Can you work these out from the model? Positions are in its coordinate system, mm. Face numbers are marked on the shaded views. A direction names the side the tool comes from. Coordinates: 2 decimals unless noted, no trailing zeros. Order: outer loops, then holes, each group sorted by start corner. A loop starts at its lowest first (then second) coordinate and runs counter-clockwise, first axis right, second up. Notation, with made-up numbers: (-31, 14.25) -> (24, 14.25) arc R16 cw to (24, 21.25) -> close; hole circle Ø9 at (72.5, 71.5). An arc over 180 degrees is marked (long way). Answer as a JSON object with one key per item and string values. Group by question number.
(1) I want a section at A-A, the plane z = 0. List the corners of the cut face in (x, y) for me, plus the area to 3 significant figures.
(2) I want a section at D-D, the plane y = -27. List the corners of the cut face in (x, z) for me, plus the area to 3 significant figures.
(3) I want a section at B-B, the plane x = 0. List the corners of the cut face in (y, z) for me, plus the area to 3 significant figures.
(4) I want a section at C-C, the plane y = -61. List the corners of the cut face in (x, z) for me, plus the area to 3 significant figures.
(5) Which directions (+Z, -Z, +X, -X, +Y, -Y) give clear straight access to the entire face, cutting with the end or side of a thin tool? Please do the marked faces 1 and 2.
(6) For pin 1 (6 mm diameter, centred on x = 5.5, y = -43, fed in from +Z); pin 2 (12 mm diameter, centred on x = 11.5, y = -39.5, fed in from +Z); pin 3 (6 mm diameter, centred on x = 10.5, y = -60, fed in from -Z), each with a flat end and sliding along its axis, tell me the tip position at first contact or that it passes through.
(7) I need wall thicknesses on line 1 (Y direction, x = 0, z = 16.5); line 2 (X direction, y = -38.5, z = -0.5) (3 decimals); line 3 (Z direction, x = 2.5, y = -6). Which ranges of each line are inside material? Lowest first, please.
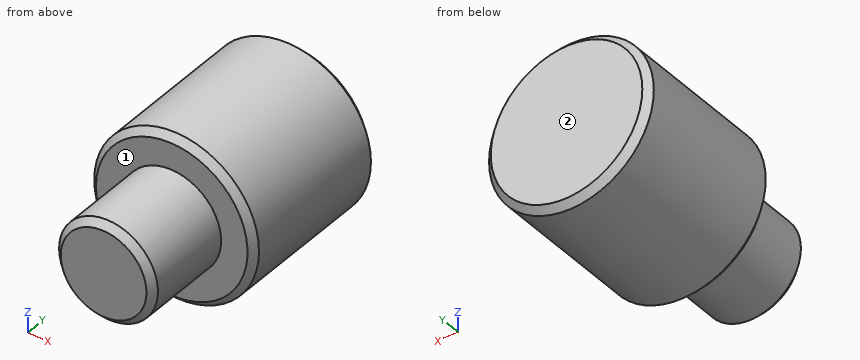
from build123d import *

# Parameters (mm, degrees)
CHAMFER1_SIZE = 2


with BuildPart() as part:
    # Sketch1 → Revolve1 (revolve)
    with BuildSketch(Plane.XY, mode=Mode.PRIVATE) as revolve1_sk:
        Polygon((0, 0), (25, 0), (25, -50), (15, -50), (15, -78), (0, -78), align=None)
    revolve(revolve1_sk.sketch.rotate(Axis((0, 5, 0), (0, -1, 0)), 180), axis=Axis((0, 5, 0), (0, -1, 0)))

    # Chamfer1
    chamfer1_edges = [part.edges().sort_by_distance(p)[0] for p in [
        (15, -78, 0),
        (25, -50, 0),
        (25, 0, 0),
    ]]
    chamfer(chamfer1_edges, length=CHAMFER1_SIZE)


solid = part.part
Computed values:
{
 "1": {"outline": "(-25, -48) -> (-23, -50) -> (-15, -50) -> (-15, -76) -> (-13, -78) -> (13, -78) -> (15, -76) -> (15, -50) -> (23, -50) -> (25, -48) -> (25, -2) -> (23, 0) -> (-23, 0) -> (-25, -2) -> close", "area": "3,330 mm2"},
 "2": {"outline": "circle Ø50 at (0, 0)", "area": "1,960 mm2"},
 "3": {"outline": "(-78, -13) -> (-76, -15) -> (-50, -15) -> (-50, -23) -> (-48, -25) -> (-2, -25) -> (0, -23) -> (0, 23) -> (-2, 25) -> (-48, 25) -> (-50, 23) -> (-50, 15) -> (-76, 15) -> (-78, 13) -> close", "area": "3,330 mm2"},
 "4": {"outline": "circle Ø30 at (0, 0)", "area": "707 mm2"},
 "5": {"face 1": "-Y", "face 2": "+Z, -Z, +X, -X, +Y"},
 "6": {"pin 1": "stops at z = 24.87", "pin 2": "stops at z = 24.39", "pin 3": "stops at z = -12.99"},
 "7": {"line 1": "y = -50 to 0", "line 2": "x = -24.995 to 24.995", "line 3": "z = -24.87 to 24.87"}
}
